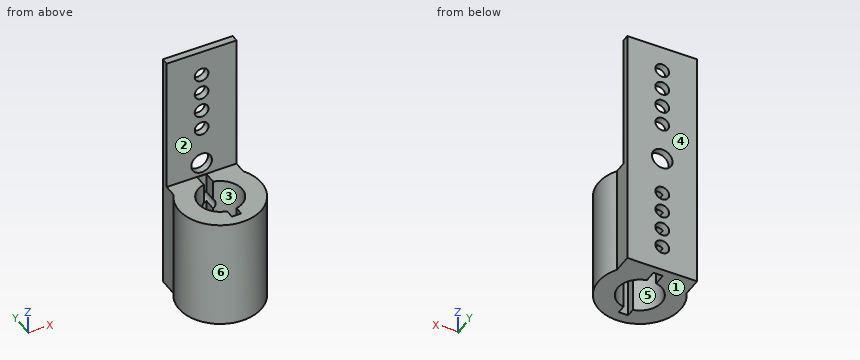
from build123d import *

# Parameters (mm, degrees)
SKETCH1_R               = 6
SKETCH1_R_2             = 3.2
BOSS_EXTRUDE1_DEPTH     = 16
SKETCH2_W               = 10.150862032
SKETCH2_H               = 2.8
BOSS_EXTRUDE2_DEPTH     = 16
CUT_EXTRUDE1_DEPTH      = 16
CUT_EXTRUDE1_DEPTH_BACK = 1
SKETCH3_W               = 1.354750416
SKETCH3_H               = 9.28691227
SKETCH4_W               = 10.150862032
SKETCH4_H               = 1.022764777
BOSS_EXTRUDE3_DEPTH     = 36
SKETCH5_R               = 1.5
CUT_EXTRUDE2_DEPTH      = 11
CUT_EXTRUDE3_DEPTH      = 11
CUT_EXTRUDE3_DEPTH_BACK = 0.1
SKETCH6_R               = 1


with BuildPart() as part:
    # Sketch1 → Boss-Extrude1 (new body)
    with BuildSketch(Plane.XY):
        Circle(SKETCH1_R)
        Circle(SKETCH1_R_2, mode=Mode.SUBTRACT)
    extrude(amount=BOSS_EXTRUDE1_DEPTH)

    # Sketch2 → Boss-Extrude2 (add)
    with BuildSketch(Plane.XY):
        with Locations((0, 4.6)):
            Rectangle(SKETCH2_W, SKETCH2_H)
    extrude(amount=BOSS_EXTRUDE2_DEPTH)

    # Sketch3 → Cut-Extrude1 (cut, two sides: drawn at the far end of the back side and taken through both)
    with BuildSketch(Plane.XY.offset(-CUT_EXTRUDE1_DEPTH_BACK)):
        with Locations((-0.009817032, 0.255242832)):
            Rectangle(SKETCH3_W, SKETCH3_H)
    extrude(amount=CUT_EXTRUDE1_DEPTH + CUT_EXTRUDE1_DEPTH_BACK, mode=Mode.SUBTRACT)

    # Sketch4 → Boss-Extrude3 (add)
    with BuildSketch(Plane.XY):
        with Locations((0, 5.488617612)):
            Rectangle(SKETCH4_W, SKETCH4_H)
    extrude(amount=BOSS_EXTRUDE3_DEPTH)

    # Sketch5 → Cut-Extrude2 (cut)
    with BuildSketch(Plane(origin=(0, 0, 0), x_dir=(1, 0, 0), z_dir=(0, 1, 0))):
        with Locations(Location((0, -18, 0), (0, 0, 90))):
            Circle(SKETCH5_R)
    extrude(amount=CUT_EXTRUDE2_DEPTH, mode=Mode.SUBTRACT)

    # Sketch6 → Cut-Extrude3 (cut, two sides: drawn at the far end of the back side and taken through both)
    with BuildSketch(Plane(origin=(0, 0, 0), x_dir=(1, 0, 0), z_dir=(0, 1, 0)).offset(-CUT_EXTRUDE3_DEPTH_BACK)):
        with Locations(Location((0, -12.4, 0), (0, 0, 90))):
            Circle(SKETCH6_R)
        with Locations(Location((0, -9.5, 0), (0, 0, 90))):
            Circle(SKETCH6_R)
        with Locations(Location((0, -6.6, 0), (0, 0, 90))):
            Circle(SKETCH6_R)
        with Locations(Location((0, -3.7, 0), (0, 0, 90))):
            Circle(SKETCH6_R)
        with Locations(Location((0, -23.6, 0), (0, 0, 90))):
            Circle(SKETCH6_R)
        with Locations(Location((0, -26.5, 0), (0, 0, 90))):
            Circle(SKETCH6_R)
        with Locations(Location((0, -29.4, 0), (0, 0, 90))):
            Circle(SKETCH6_R)
        with Locations(Location((0, -32.3, 0), (0, 0, 90))):
            Circle(SKETCH6_R)
    extrude(amount=CUT_EXTRUDE3_DEPTH + CUT_EXTRUDE3_DEPTH_BACK, mode=Mode.SUBTRACT)


solid = part.part
Geometry check sheet. Reference: the model listing, model coordinates, mm. Face numbers are marked on the shaded views. A direction names the side the tool comes from. Round coordinates to 2 decimals unless told otherwise and drop trailing zeros. Order: outer loops, then holes, each group sorted by start corner. A loop starts at its lowest first (then second) coordinate and runs counter-clockwise, first axis right, second up. Notation, with made-up numbers: M 61,21.25 L 75,21.25 A13 ccw 75,39.25 Z; hole C 68,72 d5. An arc over 180 degrees is marked long. Answer in a Markdown table with one row per item.
(1) Draft check along Y on the marked faces 3, 4, 5 and 6. Enter one of: released by +Y, released by -Y, zero draft, split by the parting line, or undercut.
Responses:
| item | result |
|---|---|
| face 3 | undercut |
| face 4 | released by +Y |
| face 5 | undercut |
| face 6 | split by the parting line |
(2) Sectioned sample at C-C, the plane z = 32.3. Record the cut outline in (x, y).
Responses:
| item | result |
|---|---|
| outline | M -5.08,4.98 L -1,4.98 L -1,6 L -5.08,6 Z; M 1,4.98 L 5.08,4.98 L 5.08,6 L 1,6 Z |
(3) Sectioned sample at B-B, the plane y = -2.75. Record the cut outline in (x, z), and give its area (3 significant figures).
Responses:
| item | result |
|---|---|
| outline | M -5.33,0 L -1.64,0 L -1.64,16 L -5.33,16 Z; M 1.64,0 L 5.33,0 L 5.33,16 L 1.64,16 Z |
| area | 118 mm² |
(4) Sectioned sample at D-D, the plane x = 0. State how many separate pieces and enclosed holes the cut face has, and give its area (3 significant figures).
Responses:
| item | result |
|---|---|
| separate pieces | 11 |
| enclosed holes | 0 |
| area | 43.8 mm² |
(5) Tool access check on the marked faces 1 and 2. Record the directions out of +Z, -Z, +X, -X, +Y, -Y that give a thin tool (end or side, any length) a straight path to the whole face; none if there is none.
Responses:
| item | result |
|---|---|
| face 1 | -Z, +X, -X, +Y, -Y |
| face 2 | +Z, +X, -X, -Y |
(6) Sectioned sample at A-A, the plane z = 14.5. Record the cut outline in (x, y), and give its area (3 significant figures).
Responses:
| item | result |
|---|---|
| outline | M -5.08,3.2 A6 ccw long 5.08,3.2 L 5.08,6 L -5.08,6 Z; hole M -0.69,-4.39 L 0.67,-4.39 L 0.67,-3.13 A3.2 ccw 0.67,3.13 L 0.67,4.9 L -0.69,4.9 L -0.69,3.13 A3.2 ccw -0.69,-3.13 Z |
| area | 85.3 mm² |
(7) Go/stop test with flat-tipped pins: P1, Ø5.5, axis at x = 0, y = -1.5, coming from the +Z side; P2, Ø1.6, axis at x = 0, z = 6.6, coming from the +Y side; P3, Ø0.7, axis at x = -0.5, z = 15, coming from the -Y side. Record where each tip stops, or that it passes through.
Responses:
| item | result |
|---|---|
| P1 | stops at z = 16 |
| P2 | stops at y = -3.1 |
| P3 | stops at y = -6 |
(8) Scan lines: probe 1 along Y at (x, z) = (0.25, 14); probe 2 along X at (y, z) = (5.7, 32.3); probe 3 along X at (y, z) = (5.25, 18). Record each from-to range of solid material in increasing order. Write a range as from..to.
Responses:
| item | result |
|---|---|
| probe 1 | y = -5.99..-4.39, 4.9..6 |
| probe 2 | x = -5.08..-1, 1..5.08 |
| probe 3 | x = -5.08..-1.5, 1.5..5.08 |
